Part model, mm, in its own coordinate system. Face numbers are marked on the shaded views. A direction names the side the tool comes from. Give positions to 0.01 mm unless a question says otherwise; leave off trailing zeros. Order: outer loops, then holes, each group sorted by start corner. A loop starts at its lowest first (then second) coordinate and runs counter-clockwise, first axis right, second up. Notation, with made-up numbers: (47.5, -39) - (59.5, -39) arc R8 cw to (59.5, -31) - close; hole circle Ø6 at (47, 49). An arc over 180 degrees is marked (long way). One line per item, written item: value.
```python
from build123d import *

# Parameters (mm, degrees)
F1_DEPTH        = 10
F0_R            = 2.9
F2_DEPTH        = 3
F3_R            = 6.5
F4_DEPTH        = 4
F5_R            = 5
F6_DEPTH        = 12
F7_DEPTH        = 2
F8_D            = 3.3
F8_DEPTH        = 13.8
F8_START        = 2
F8_TIP          = 0.9914200214
F9_DEPTH        = 1.4
F10_D           = 3.3
F10_DEPTH       = 8
F10_TIP         = 0.9914200214
F12_D           = 3.3
F12_DEPTH       = 8
F12_CSINK_D     = 6.72
F12_CSINK_ANGLE = 90
F12_TIP         = 0.9914200214


with BuildPart() as f1:
    # F0 (on Front) → F1 (new body)
    with BuildSketch(Plane.XZ):
        with BuildLine():
            Line((20.9, 37.9), (17.9, 37.9))
            Line((17.9, 37.9), (-17.9, 37.9))
            Line((-17.9, 37.9), (-20.9, 37.9))
            ThreePointArc((-20.9, 37.9), (-22.3142135624, 37.3142135624), (-22.9, 35.9))
            Line((-22.9, 35.9), (-22.9, 32.9))
            Line((-22.9, 32.9), (-22.9, -35.9))
            ThreePointArc((-22.9, -35.9), (-22.3142135624, -37.3142135624), (-20.9, -37.9))
            Line((-20.9, -37.9), (20.9, -37.9))
            ThreePointArc((20.9, -37.9), (22.3142135624, -37.3142135624), (22.9, -35.9))
            Line((22.9, -35.9), (22.9, 32.9))
            Line((22.9, 32.9), (22.9, 35.9))
            ThreePointArc((22.9, 35.9), (22.3142135624, 37.3142135624), (20.9, 37.9))
        make_face()
        Polygon((7.4256842194, -31), (10.7743157806, -31), (12.4486315613, -33.9), (10.7743157806, -36.8), (7.4256842194, -36.8), (5.7513684387, -33.9), align=None, mode=Mode.SUBTRACT)
        Polygon((-16.2256842194, 36.8), (-14.5513684387, 33.9), (-16.2256842194, 31), (-19.5743157806, 31), (-21.2486315613, 33.9), (-19.5743157806, 36.8), align=None, mode=Mode.SUBTRACT)
        Polygon((20.9, 29.9), (20.9, -29.9), (18.3, -29.9), (-18.8811943151, -29.9), (-20.9, -29.9), (-20.9, 29.9), align=None, mode=Mode.SUBTRACT)
        Polygon((21.2486315613, 33.9), (19.5743157806, 31), (16.2256842194, 31), (14.5513684387, 33.9), (16.2256842194, 36.8), (19.5743157806, 36.8), align=None, mode=Mode.SUBTRACT)
        Polygon((-16.2256842194, 31), (-14.5513684387, 33.9), (-16.2256842194, 36.8), (-19.5743157806, 36.8), (-21.2486315613, 33.9), (-19.5743157806, 31), align=None)
        Polygon((16.2256842194, 31), (19.5743157806, 31), (21.2486315613, 33.9), (19.5743157806, 36.8), (16.2256842194, 36.8), (14.5513684387, 33.9), align=None)
        Polygon((12.4486315613, -33.9), (10.7743157806, -31), (7.4256842194, -31), (5.7513684387, -33.9), (7.4256842194, -36.8), (10.7743157806, -36.8), align=None)
    extrude(amount=F1_DEPTH)

    # F0 (on Front) → F2 (join)
    with BuildSketch(Plane.XZ):
        with BuildLine():
            Line((18.3, -29.9), (20.9, -29.9))
            Line((20.9, -29.9), (20.9, 29.9))
            Line((20.9, 29.9), (-20.9, 29.9))
            Line((-20.9, 29.9), (-20.9, -29.9))
            Line((-20.9, -29.9), (-18.8811943151, -29.9))
            Line((-18.8811943151, -29.9), (-18.8811943151, -20.7887917079))
            ThreePointArc((-18.8811943151, -20.7887917079), (-18.7640370276, -20.5059489954), (-18.4811943151, -20.3887917079))
            Line((-18.4811943151, -20.3887917079), (-17.9, -20.3887917079))
            ThreePointArc((-17.9, -20.3887917079), (-17.1928932188, -20.0958984891), (-16.9, -19.3887917079))
            Line((-16.9, -19.3887917079), (-16.9, -13))
            ThreePointArc((-16.9, -13), (-16.0213203436, -10.8786796564), (-13.9, -10))
            Line((-13.9, -10), (13.9, -10))
            ThreePointArc((13.9, -10), (16.0213203436, -10.8786796564), (16.9, -13))
            Line((16.9, -13), (16.9, -19.3887917079))
            ThreePointArc((16.9, -19.3887917079), (17.1928932188, -20.0958984891), (17.9, -20.3887917079))
            ThreePointArc((17.9, -20.3887917079), (18.1828427125, -20.5059489954), (18.3, -20.7887917079))
            Line((18.3, -20.7887917079), (18.3, -29.9))
        make_face()
        with Locations((-8.5, 0)):
            Circle(F0_R, mode=Mode.SUBTRACT)
        with Locations((8.5, 0)):
            Circle(F0_R, mode=Mode.SUBTRACT)
        with BuildLine():
            ThreePointArc((-16.9, 23.6416198403), (-16.0213203436, 25.7629401838), (-13.9, 26.6416198403))
            Line((-13.9, 26.6416198403), (13.9, 26.6416198403))
            ThreePointArc((13.9, 26.6416198403), (16.0213203436, 25.7629401838), (16.9, 23.6416198403))
            Line((16.9, 23.6416198403), (16.9, 13))
            ThreePointArc((16.9, 13), (16.0213203436, 10.8786796564), (13.9, 10))
            Line((13.9, 10), (-13.9, 10))
            ThreePointArc((-13.9, 10), (-16.0213203436, 10.8786796564), (-16.9, 13))
            Line((-16.9, 13), (-16.9, 23.6416198403))
        make_face(mode=Mode.SUBTRACT)
        with Locations((-8.5, 0)):
            Circle(F0_R)
        with Locations((8.5, 0)):
            Circle(F0_R)
    extrude(amount=F2_DEPTH)

    # F3 (on face) → F4 (cut)
    with BuildSketch(Plane.YZ.offset(22.9)):
        with Locations((-13.5, 17.9)):
            Circle(F3_R)
    extrude(amount=-F4_DEPTH, mode=Mode.SUBTRACT)

    # F5 (on face) → F6 (cut)
    with BuildSketch(Plane.XY.offset(37.9)):
        with Locations((-10.8651584014, -13)):
            Circle(F5_R)
    extrude(amount=-F6_DEPTH, mode=Mode.SUBTRACT)

    # F0 (on Front) → F7 (cut)
    with BuildSketch(Plane.XZ):
        Polygon((-16.2256842194, 31), (-14.5513684387, 33.9), (-16.2256842194, 36.8), (-19.5743157806, 36.8), (-21.2486315613, 33.9), (-19.5743157806, 31), align=None)
        Polygon((16.2256842194, 31), (19.5743157806, 31), (21.2486315613, 33.9), (19.5743157806, 36.8), (16.2256842194, 36.8), (14.5513684387, 33.9), align=None)
        Polygon((12.4486315613, -33.9), (10.7743157806, -31), (7.4256842194, -31), (5.7513684387, -33.9), (7.4256842194, -36.8), (10.7743157806, -36.8), align=None)
    extrude(amount=F7_DEPTH, mode=Mode.SUBTRACT)

    # F8
    # its depths count from where the whole tool has entered the part; down to there all is cleared
    with Locations(Plane(origin=(0, 0, 0), x_dir=(1, 0, 0), z_dir=(0, 1, 0)).offset(-F8_START)):
        with Locations((-17.9, -33.9), (17.9, -33.9), (9.1, 33.9)):
            Hole(F8_D / 2, depth=F8_DEPTH)
            with Locations((0, 0, -(F8_DEPTH + F8_TIP / 2))):  # 118° drill point
                Cone(0, F8_D / 2, F8_TIP, mode=Mode.SUBTRACT)

    # F0 (on Front) → F9 (join)
    with BuildSketch(Plane.XZ):
        with Locations((8.5, 0)):
            Circle(F0_R)
        with Locations((-8.5, 0)):
            Circle(F0_R)
    extrude(amount=-F9_DEPTH)

    # F10 (one way)
    with BuildSketch(Plane.XZ):
        with Locations((-8.5, 0), (8.5, 0)):
            Circle(F10_D / 2)
    extrude(amount=-F10_DEPTH, mode=Mode.SUBTRACT)
    with Locations(Plane.XZ):
        with Locations((-8.5, 0), (8.5, 0)):
            with Locations((0, 0, -(F10_DEPTH + F10_TIP / 2))):  # 118° drill point
                Cone(0, F10_D / 2, F10_TIP, mode=Mode.SUBTRACT)

    # F12
    with Locations(Plane.XZ.offset(3)):
        with Locations((-8.5, 0), (8.5, 0)):
            CounterSinkHole(F12_D / 2, F12_CSINK_D / 2, depth=F12_DEPTH, counter_sink_angle=F12_CSINK_ANGLE)
            with Locations((0, 0, -(F12_DEPTH + F12_TIP / 2))):  # 118° drill point
                Cone(0, F12_D / 2, F12_TIP, mode=Mode.SUBTRACT)


solid = f1.part
```
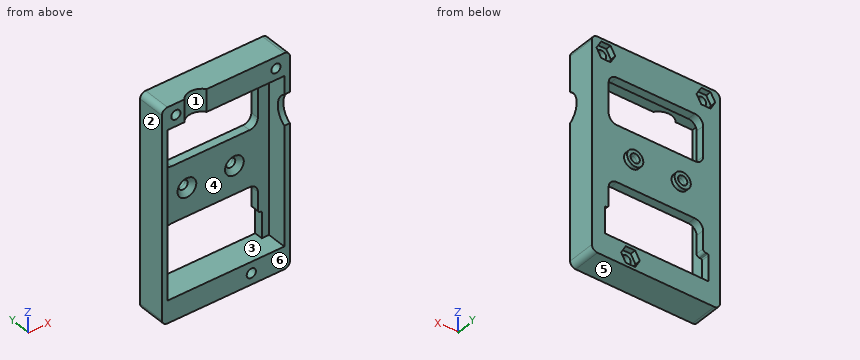
1) Cut at C-C, the plane z = 7. Give the cut face in (x, y).
Outcome:
outline: (-22.9, -10) - (-20.9, -10) - (-20.9, -3) - (20.9, -3) - (20.9, -10) - (22.9, -10) - (22.9, 0) - (-22.9, 0) - close
2) Which spindle directions (+Z, -Z, +X, -X, +Y, -Y) get a long thin tool onto all of the face, cutting with end or side? Do the marked faces 1 and 2. Say none if no direction does.
Outcome:
face 1: +Z, -Y
face 2: +Z, -Z, -X, +Y, -Y
3) Mould opens along Z. For the marked faces 3, 4, 5 and 6 say: released by +Z, released by -Z, zero draft, split by the parting line, or undercut.
Outcome:
face 3: undercut
face 4: undercut
face 5: released by -Z
face 6: zero draft
4) Cut at B-B, the plane z = -29. Give the cut face in (x, y).
Outcome:
outline: (-22.9, -10) - (-20.9, -10) - (-20.9, -3) - (-18.88, -3) - (-18.88, 0) - (-22.9, 0) - close; (18.3, -3) - (20.9, -3) - (20.9, -10) - (22.9, -10) - (22.9, 0) - (18.3, 0) - close
5) Pin check, flat tips, straight feed: pin 1 (4.5 mm diameter, centred on x = -16.5, z = 32.5, fed in from +Y); pin 2 (1.7 mm diameter, centred on x = 7.5, z = -33.5, fed in from +Y); pin 3 (2 mm diameter, centred on x = 8.5, z = 0, fed in from -Y) (1 decimal). Stop position of each tip, or through.
Outcome:
pin 1: stops at y = 0
pin 2: stops at y = -2
pin 3: passes through
6) Drill centre lines: line 1 along Z through (x, y) = (17.9, -4); line 2 along Z through (x, y) = (9.1, -5.5); line 3 along X through (y, z) = (-0.55, 0). Where is each one in solid material? Low to high. Write a range as from..to.
Outcome:
line 1: z = -37.9..-29.9, 29.9..32.25, 35.55..37.9
line 2: z = -37.9..-35.55, -32.25..-29.9, 29.9..37.9
line 3: x = -22.9..-10.15, -6.85..6.85, 10.15..22.9
7) Cut at A-A, the plane y = -4.5. Give the cut face in (x, z).
Outcome:
outline: (-22.9, -35.9) arc R2 ccw to (-20.9, -37.9) - (20.9, -37.9) arc R2 ccw to (22.9, -35.9) - (22.9, 35.9) arc R2 ccw to (20.9, 37.9) - (-20.9, 37.9) arc R2 ccw to (-22.9, 35.9) - close; hole (-20.9, -29.9) - (20.9, -29.9) - (20.9, 29.9) - (-20.9, 29.9) - close; hole circle Ø3.3 at (-17.9, 33.9); hole circle Ø3.3 at (9.1, -33.9); hole circle Ø3.3 at (17.9, 33.9)
8) Cut at D-D, the plane x = 8.5. Give the number of separate pieces and of enclosed holes in the cut face, then the cut area to 3 significant figures.
Outcome:
separate pieces: 5
enclosed holes: 0
area: 184 mm^2
